Can you work these out from the model? Positions are in its coordinate system, mm. Face numbers are marked on the shaded views. A direction names the side the tool comes from. Give positions to 0.01 mm unless a question says otherwise; leave off trailing zeros. Loops run counter-clockwise (first coordinate to the right, second up) from the corner with the lowest first, then second, coordinate; pieces in that order, holes last. Notation, with made-up numbers: M -20.75,-3 L 37.25,-3 A31 ccw 37.25,26 Z; hole C -10,59 d7. An arc over 180 degrees is marked long. One line per item, written item: value. Start each with the question number.
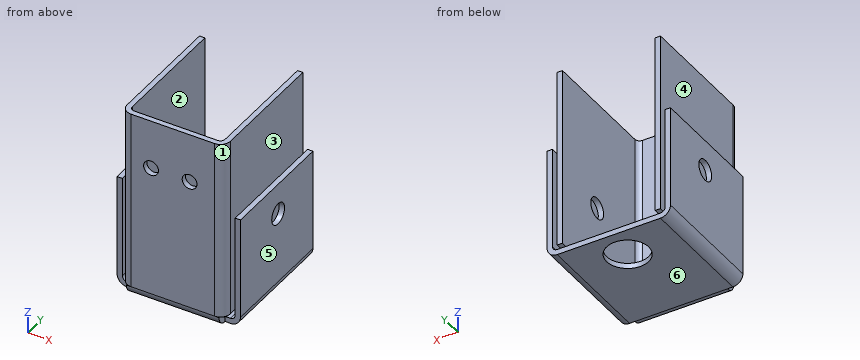
from build123d import *

# Parameters (mm, degrees)
SKETCH1_W                    = 15
SKETCH1_H                    = 30
BASE_FLANGE1_DEPTH           = 0.86
EDGE_FLANGE1_STRIP_W         = 4.964
EDGE_FLANGE1_STRIP_H         = 0.86
EDGE_FLANGE1_STRIP_CUT_DEPTH = 15
EDGE_FLANGE1_DEPTH           = 15
EDGE_FLANGE2_STRIP_W         = 4.964
EDGE_FLANGE2_STRIP_H         = 0.86
EDGE_FLANGE2_STRIP_CUT_DEPTH = 29.238
EDGE_FLANGE2_DEPTH           = 29.238
EDGE_FLANGE3_STRIP_W         = 4.964
EDGE_FLANGE3_STRIP_H         = 0.86
EDGE_FLANGE3_STRIP_CUT_DEPTH = 29.238
EDGE_FLANGE3_DEPTH           = 29.238
EDGE_FLANGE4_START           = 0.762
EDGE_FLANGE4_DEPTH           = 19.238
EDGE_FLANGE5_START           = 0.762
EDGE_FLANGE5_DEPTH           = 19.238
SKETCH21_R                   = 3.4
CUT_EXTRUDE1_DEPTH           = 10
M3_CLEARANCE_HOLE2_D         = 3.4
M2_CLEARANCE_HOLE1_D         = 2.4
M2_CLEARANCE_HOLE1_DEPTH     = 12
M2_CLEARANCE_HOLE1_TIP       = 0.721032743


# Read off the part's stored shape, not the designer's step: Edge-Flange4, Edge-Flange5
# Sheet-metal steps are written as plain solids
with BuildPart() as part:
    # Sketch1 → Base-Flange1 (new body)
    with BuildSketch(Plane(origin=(0, 0, 0), x_dir=(1, 0, 0), z_dir=(0, 1, 0))):
        Rectangle(SKETCH1_W, SKETCH1_H)
    extrude(amount=-BASE_FLANGE1_DEPTH)

    # Edge-Flange1 strip (across the edge) → Edge-Flange1 strip cut (cut)
    with BuildSketch(Plane(origin=(7.5, 0, -15), x_dir=(0, 0, 1), z_dir=(-1, 0, 0))):
        with Locations((-1.72, -0.43)):
            Rectangle(EDGE_FLANGE1_STRIP_W, EDGE_FLANGE1_STRIP_H)
    extrude(amount=EDGE_FLANGE1_STRIP_CUT_DEPTH, mode=Mode.SUBTRACT)

    # Edge-Flange1 section (across the edge) → Edge-Flange1 (add)
    with BuildSketch(Plane(origin=(7.5, 0, -15), x_dir=(0, 0, 1), z_dir=(-1, 0, 0))):
        with BuildLine():
            Line((-0.86, 0.762), (-0.86, 20))
            Line((-0.86, 20), (0, 20))
            Line((0, 20), (0, 0.762))
            ThreePointArc((0, 0.762), (0.223184633, 0.223184633), (0.762, 0))
            Line((0.762, 0), (0.762, -0.86))
            ThreePointArc((0.762, -0.86), (-0.384927199, -0.384927199), (-0.86, 0.762))
        make_face()
    extrude(amount=EDGE_FLANGE1_DEPTH)

    # Edge-Flange2 strip (across the edge) → Edge-Flange2 strip cut (cut)
    with BuildSketch(Plane(origin=(7.5, 0, 15), x_dir=(-1, 0, 0), z_dir=(0, 0, -1))):
        with Locations((-1.72, -0.43)):
            Rectangle(EDGE_FLANGE2_STRIP_W, EDGE_FLANGE2_STRIP_H)
    extrude(amount=EDGE_FLANGE2_STRIP_CUT_DEPTH, mode=Mode.SUBTRACT)

    # Edge-Flange2 section (across the edge) → Edge-Flange2 (add)
    with BuildSketch(Plane(origin=(7.5, 0, 15), x_dir=(-1, 0, 0), z_dir=(0, 0, -1))):
        with BuildLine():
            Line((-0.86, 0.762), (-0.86, 20))
            Line((-0.86, 20), (0, 20))
            Line((0, 20), (0, 0.762))
            ThreePointArc((0, 0.762), (0.223184633, 0.223184633), (0.762, 0))
            Line((0.762, 0), (0.762, -0.86))
            ThreePointArc((0.762, -0.86), (-0.384927199, -0.384927199), (-0.86, 0.762))
        make_face()
    extrude(amount=EDGE_FLANGE2_DEPTH)

    # Edge-Flange3 strip (across the edge) → Edge-Flange3 strip cut (cut)
    with BuildSketch(Plane(origin=(-7.5, 0, -14.238), x_dir=(1, 0, 0), z_dir=(0, 0, 1))):
        with Locations((-1.72, -0.43)):
            Rectangle(EDGE_FLANGE3_STRIP_W, EDGE_FLANGE3_STRIP_H)
    extrude(amount=EDGE_FLANGE3_STRIP_CUT_DEPTH, mode=Mode.SUBTRACT)

    # Edge-Flange3 section (across the edge) → Edge-Flange3 (add)
    with BuildSketch(Plane(origin=(-7.5, 0, -14.238), x_dir=(1, 0, 0), z_dir=(0, 0, 1))):
        with BuildLine():
            Line((-0.86, 0.762), (-0.86, 20))
            Line((-0.86, 20), (0, 20))
            Line((0, 20), (0, 0.762))
            ThreePointArc((0, 0.762), (0.223184633, 0.223184633), (0.762, 0))
            Line((0.762, 0), (0.762, -0.86))
            ThreePointArc((0.762, -0.86), (-0.384927199, -0.384927199), (-0.86, 0.762))
        make_face()
    extrude(amount=EDGE_FLANGE3_DEPTH)

    # Edge-Flange4 outline → Edge-Flange4 (add)
    with BuildSketch(Plane(origin=(0, 0, 0), x_dir=(1, 0, 0), z_dir=(0, 1, 0)).offset(EDGE_FLANGE4_START)):
        with BuildLine():
            ThreePointArc((-8.36, 15.86), (-9.506927199, 15.384927199), (-9.982, 14.238))
            Line((-9.982, 14.238), (-9.982, -2.25))
            Line((-9.982, -2.25), (-9.122, -2.25))
            Line((-9.122, -2.25), (-9.122, 14.238))
            ThreePointArc((-9.122, 14.238), (-8.898815367, 14.776815367), (-8.36, 15))
            Line((-8.36, 15), (-7.5, 15))
            Line((-7.5, 15), (-7.5, 15.86))
            Line((-7.5, 15.86), (-8.36, 15.86))
        make_face()
    extrude(amount=EDGE_FLANGE4_DEPTH)

    # Edge-Flange5 outline → Edge-Flange5 (add)
    with BuildSketch(Plane(origin=(0, 0, 0), x_dir=(1, 0, 0), z_dir=(0, 1, 0)).offset(EDGE_FLANGE5_START)):
        with BuildLine():
            Line((9.122, -2.25), (9.982, -2.25))
            Line((9.982, -2.25), (9.982, 14.238))
            ThreePointArc((9.982, 14.238), (9.506927199, 15.384927199), (8.36, 15.86))
            Line((8.36, 15.86), (7.5, 15.86))
            Line((7.5, 15.86), (7.5, 15))
            Line((7.5, 15), (8.36, 15))
            ThreePointArc((8.36, 15), (8.898815367, 14.776815367), (9.122, 14.238))
            Line((9.122, 14.238), (9.122, -2.25))
        make_face()
    extrude(amount=EDGE_FLANGE5_DEPTH)

    # Sketch21 → Cut-Extrude1 (cut)
    with BuildSketch(Plane(origin=(0, 0, -15.86), x_dir=(-1, 0, 0), z_dir=(0, 0, -1))):
        with Locations(Location((0, 15, 0), (0, 0, 90))):
            Circle(SKETCH21_R)
    extrude(amount=-CUT_EXTRUDE1_DEPTH, mode=Mode.SUBTRACT)

    # M3 Clearance Hole2 (through all)
    with Locations(Plane.ZY.offset(9.982)):
        with Locations((-2.75, 10.762)):
            Hole(M3_CLEARANCE_HOLE2_D / 2)

    # M2 Clearance Hole1
    with Locations(Plane(origin=(0, 0, 0), x_dir=(1, 0, 0), z_dir=(0, 1, 0))):
        with Locations((2.738, -7.031765706), (-3.5, -7.031765706)):
            Hole(M2_CLEARANCE_HOLE1_D / 2, depth=M2_CLEARANCE_HOLE1_DEPTH)
            with Locations((0, 0, -(M2_CLEARANCE_HOLE1_DEPTH + M2_CLEARANCE_HOLE1_TIP / 2))):  # 118° drill point
                Cone(0, M2_CLEARANCE_HOLE1_D / 2, M2_CLEARANCE_HOLE1_TIP, mode=Mode.SUBTRACT)


solid = part.part
Q1. If we section it at C-C, the plane y = 3.25: Write out the boundary of the cut face in (x, z), plus the area to 3 significant figures.
Q2. If we section it at A-A, the plane z = -7.5: Write out the boundary of the cut face in (x, y).
Q3. Which directions (+Z, -Z, +X, -X, +Y, -Y) give clear straight access to the entire face, cutting with the end or side of a thin tool? Please do the marked faces 1, 2 and 3.
Q4. If we section it at B-B, the plane x = 5: Write out the boundary of the cut face in (y, z).
Q5. If we section it at D-D, the plane y = 15: Write out the boundary of the cut face in (x, z).
Q6. If we mould it in two halves opening along X, with no side actions, what happens to the marked faces 4, 5 and 6? For each: released by +X, released by -X, zero draft, split by the parting line, or undercut.
Q7. I need wall thicknesses on line 1 along X through (y, z) = (8.75, -11.5); line 2 along Y through (x, z) = (-9.65, -2.75); line 3 along X through (y, z) = (2.5, 7). Which ranges of each line are inside material? Lowest first, please.
Q8. For P1, Ø4, axis at x = -1, y = 13, coming from the +Z side; P2, Ø2, axis at y = 6.5, z = 7, coming from the +X side; P3, Ø2.5, axis at y = 10.762, z = -2.75, coming from the -X side; P4, Ø4, axis at x = 2.74, z = 7.03, coming from the +Y side, each with a flat end and sliding along its axis, tell me the tip position at first contact or that it passes through.
Response:
1. outline: M -9.98,-14.24 A1.62 ccw -8.36,-15.86 L 8.36,-15.86 A1.62 ccw 9.98,-14.24 L 9.98,2.25 L 9.12,2.25 L 9.12,-14.24 A0.76 cw 8.36,-15 L -8.36,-15 A0.76 cw -9.12,-14.24 L -9.12,2.25 L -9.98,2.25 Z; M -8.36,-14.24 L -7.5,-14.24 L -7.5,15 L -8.36,15 Z; M 7.5,-14.24 L 8.36,-14.24 L 8.36,15 L 7.5,15 Z
1. area: 96.2 mm^2
2. outline: M -9.98,0.76 L -9.12,0.76 L -9.12,20 L -9.98,20 Z; M -8.36,0.76 A1.62 ccw -6.74,-0.86 L 6.74,-0.86 A1.62 ccw 8.36,0.76 L 8.36,20 L 7.5,20 L 7.5,0.76 A0.76 cw 6.74,0 L -6.74,0 A0.76 cw -7.5,0.76 L -7.5,20 L -8.36,20 Z; M 9.12,0.76 L 9.98,0.76 L 9.98,20 L 9.12,20 Z
3. face 1: +Z, +X, -Y
3. face 2: +Z, +Y
3. face 3: +Z, +Y, -Y
4. outline: M -0.86,-14.24 A1.62 ccw 0.76,-15.86 L 20,-15.86 L 20,-15 L 0.76,-15 A0.76 cw 0,-14.24 L 0,15 L -0.86,15 Z
5. outline: M -9.98,-14.24 A1.62 ccw -8.36,-15.86 L -3.4,-15.86 L -3.4,-15 L -8.36,-15 A0.76 cw -9.12,-14.24 L -9.12,2.25 L -9.98,2.25 Z; M -8.36,-14.24 L -7.5,-14.24 L -7.5,15 L -8.36,15 Z; M 3.4,-15.86 L 8.36,-15.86 A1.62 ccw 9.98,-14.24 L 9.98,2.25 L 9.12,2.25 L 9.12,-14.24 A0.76 cw 8.36,-15 L 3.4,-15 Z; M 7.5,-14.24 L 8.36,-14.24 L 8.36,15 L 7.5,15 Z
6. face 4: undercut
6. face 5: released by +X
6. face 6: zero draft
7. line 1: -9.98 to -9.12, -8.36 to -7.5, 7.5 to 8.36, 9.12 to 9.98
7. line 2: 0.76 to 9.06, 12.46 to 20
7. line 3: -8.36 to -7.5, 7.5 to 8.36
8. P1: z = -15
8. P2: x = 8.36
8. P3: through
8. P4: y = 0
